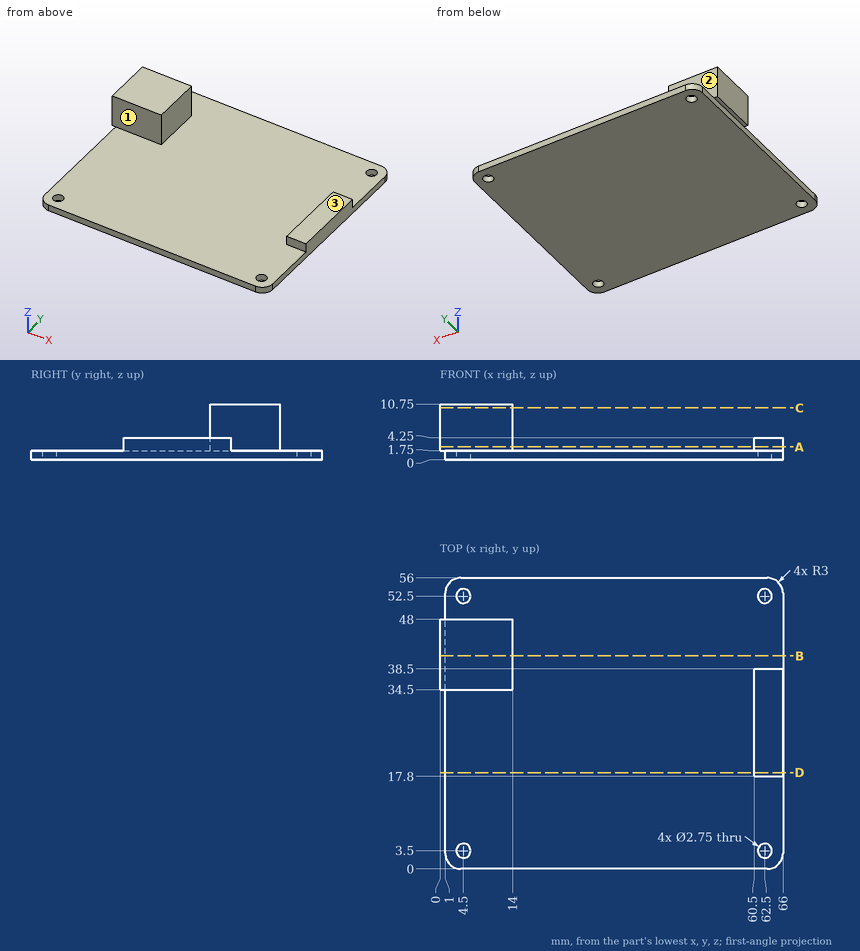
Source: three-view drawing plus pictorial views. Frame: mm from the lowest corner of the part. A direction names the side the tool comes from. Give positions to 0.01 mm unless a question says otherwise; leave off trailing zeros. Order: outer loops, then holes, each group sorted by start corner. A loop starts at its lowest first (then second) coordinate and runs counter-clockwise, first axis right, second up. Notation, with made-up numbers: (47.5, -21.5) - (85.5, -21.5) arc R6 ccw to (85.5, -17.5) - close; hole circle Ø3 at (-2, 8.25). An arc over 180 degrees is marked (long way). Answer as a JSON object with one key per item and string values. Group by question number.
Q1. Cut plane A-A, the plane z = 2.5. Output: boundary loops of the cut face in (x, y).
Q2. Line query: probe 1 along X at (y, z) = (52.5, 0.55) (3 decimals); probe 2 along Y at (x, z) = (4.5, 0.9) (3 decimals); probe 3 along X at (y, z) = (3, 1). Output: solid intervals per line, ascending.
Q3. Cut plane C-C, the plane z = 10. Output: boundary loops of the cut face in (x, y).
Q4. Cut plane D-D, the plane y = 18.5. Output: boundary loops of the cut face in (x, z).
Q5. Cut plane B-B, the plane y = 41. Output: boundary loops of the cut face in (x, z).
Q6. First-contact query: pin 1 Ø1.9 at (y, z) = (36, 1) entering from -X; pin 2 Ø0.8 at (x, z) = (63.5, 2.5) entering from +Y; pin 3 Ø3 at (y, z) = (50, 4.5) entering from -X; pin 4 Ø6 at (x, y) = (63, 26) entering from +Z. Flat tips, straight axial feed; report the tip coordinate or a pass-through.
Q7. Set-up query: the marked faces 1, 2 and 3. Return all of +Z, -Z, +X, -X, +Y, -Y with unobstructed straight access to the full face (end or side cutting, diameter ignored); none if empty.
Results:
{
 "1": {"outline": "(0, 34.5) - (14, 34.5) - (14, 48) - (0, 48) - close; (60.5, 17.8) - (66, 17.8) - (66, 38.5) - (60.5, 38.5) - close"},
 "2": {"probe 1": "1 to 3.125, 5.875 to 61.125, 63.875 to 66", "probe 2": "0 to 2.125, 4.875 to 51.125, 53.875 to 56", "probe 3": "1 to 3.22, 5.78 to 61.22, 63.78 to 66"},
 "3": {"outline": "(0, 34.5) - (14, 34.5) - (14, 48) - (0, 48) - close"},
 "4": {"outline": "(1, 0) - (66, 0) - (66, 4.25) - (60.5, 4.25) - (60.5, 1.75) - (1, 1.75) - close"},
 "5": {"outline": "(0, 1.75) - (1, 1.75) - (1, 0) - (66, 0) - (66, 1.75) - (14, 1.75) - (14, 10.75) - (0, 10.75) - close"},
 "6": {"pin 1": "x = 0", "pin 2": "y = 38.5", "pin 3": "through", "pin 4": "z = 4.25"},
 "7": {"face 1": "+Z, -X, -Y", "face 2": "+Z, +X, -X, +Y", "face 3": "+Z, +X, +Y, -Y"}
}
